from build123d import *

# Parameters (mm, degrees)
SKETCH1_W           = 120
SKETCH1_H           = 43
SKETCH1_R           = 2.075
SKETCH1_R_2         = 2.05
SKETCH1_R_3         = 7
BOSS_EXTRUDE1_DEPTH = 3.125
FILLET1_R           = 5


with BuildPart() as part:
    # Sketch1 → Boss-Extrude1 (new body)
    with BuildSketch(Plane.XY):
        Rectangle(SKETCH1_W, SKETCH1_H)
        with Locations((-52, 16)):
            Circle(SKETCH1_R, mode=Mode.SUBTRACT)
        with Locations((-52, -16)):
            Circle(SKETCH1_R, mode=Mode.SUBTRACT)
        with Locations((28, 8)):
            Circle(SKETCH1_R_2, mode=Mode.SUBTRACT)
        with Locations((44, 8)):
            Circle(SKETCH1_R_2, mode=Mode.SUBTRACT)
        with Locations((44, -8)):
            Circle(SKETCH1_R_2, mode=Mode.SUBTRACT)
        with Locations((36, 0)):
            Circle(SKETCH1_R_3, mode=Mode.SUBTRACT)
        with Locations((28, -8)):
            Circle(SKETCH1_R_2, mode=Mode.SUBTRACT)
    extrude(amount=BOSS_EXTRUDE1_DEPTH)

    # Fillet1
    fillet1_edges = [part.edges().sort_by_distance(p)[0] for p in [
        (-60, 21.5, 1.5625),
        (60, 21.5, 1.5625),
        (60, -21.5, 1.5625),
        (-60, -21.5, 1.5625),
    ]]
    fillet(fillet1_edges, radius=FILLET1_R)


solid = part.part
For this review, take the finished solid that the model builds, in its own axes (mm). Give positions to 0.01 mm unless a question says otherwise; leave off trailing zeros. Loops run counter-clockwise (first coordinate to the right, second up) from the corner with the lowest first, then second, coordinate; pieces in that order, holes last. Notation, with made-up numbers: (18, 61.25) - (67, 61.25) arc R19 ccw to (67, 81.25) - close; hole circle Ø10 at (-11.75, 58.25). An arc over 180 degrees is marked (long way). Write each question's results on one line, items separated by ' | '.
(1) Draft analysis for pull direction Y (two halves, no side actions). For faces 1 (the flat face through (-1, 0, 3.125)), 2 (the cylindrical face through (-58.57, 20, 1.58)), 3 (the cylindrical face through (41.95, -7.91, 1.54)), state which applies: +Y half, -Y half, draft (parallel to the pull), parting line (faces both ways), or undercut.
Conclusion:
face 1: draft | face 2: +Y half | face 3: undercut
(2) Take a section at C-C (z = 1.35). Give the boundary of the cut face in (x, y) (3 decimals).
Conclusion:
outline: (-60, -16.5) arc R5 ccw to (-55, -21.5) - (55, -21.5) arc R5 ccw to (60, -16.5) - (60, 16.5) arc R5 ccw to (55, 21.5) - (-55, 21.5) arc R5 ccw to (-60, 16.5) - close; hole circle Ø4.15 at (-52, -16); hole circle Ø4.15 at (-52, 16); hole circle Ø4.1 at (28, -8); hole circle Ø4.1 at (28, 8); hole circle Ø14 at (36, 0); hole circle Ø4.1 at (44, -8); hole circle Ø4.1 at (44, 8)
(3) Take a section at B-B (x = -52). Give the boundary of the cut face in (y, z) (3 decimals).
Conclusion:
outline: (-21.5, 0) - (-18.075, 0) - (-18.075, 3.125) - (-21.5, 3.125) - close; (-13.925, 0) - (13.925, 0) - (13.925, 3.125) - (-13.925, 3.125) - close; (18.075, 0) - (21.5, 0) - (21.5, 3.125) - (18.075, 3.125) - close
(4) Take a section at D-D (x = 38). Give the boundary of the cut face in (y, z) (3 decimals).
Conclusion:
outline: (-21.5, 0) - (-6.708, 0) - (-6.708, 3.125) - (-21.5, 3.125) - close; (6.708, 0) - (21.5, 0) - (21.5, 3.125) - (6.708, 3.125) - close
(5) For line 1 along Y through (x, z) = (44, 0.65); line 2 along X through (y, z) = (-2.5, 2.6); line 3 along X through (y, z) = (1.5, 0.2), list the stretches that pass through material, from the lowest coordinate up.
Conclusion:
line 1: -21.5 to -10.05, -5.95 to 5.95, 10.05 to 21.5 | line 2: -60 to 29.46, 42.54 to 60 | line 3: -60 to 29.16, 42.84 to 60
(6) For pin 1 Ø3.5 at (x, y) = (44, -8) entering from +Z, flat-tipped, find the tip position at first contact; note if it passes through.
Conclusion:
pin 1: through
(7) Take a section at A-A (y = 0). Give the boundary of the cut face in (x, z) (3 decimals).
Conclusion:
outline: (-60, 0) - (29, 0) - (29, 3.125) - (-60, 3.125) - close; (43, 0) - (60, 0) - (60, 3.125) - (43, 3.125) - close
